Source: CAD feature listing. Evaluate the final solid. Frame: model axes, mm. A direction names the side the tool comes from. Round coordinates to 2 decimals unless told otherwise and drop trailing zeros. Order: outer loops, then holes, each group sorted by start corner. A loop starts at its lowest first (then second) coordinate and runs counter-clockwise, first axis right, second up. Notation, with made-up numbers: M 75.5,-38 L 101.5,-38 A6 ccw 101.5,-28 Z; hole C -28.75,52.25 d5. An arc over 180 degrees is marked long. Use one line per item in the form item = value. Start each with the question number.
Q1. Reachability of faces 1 (the cylindrical face through (-567.96, -22, 0.51)), 2 (the flat face through (-646.372, -29.58, 0.746)), 3 (the flat face through (-8.872, -30.42, 0.746)) from +Z, -Z, +X, -X, +Y, -Y: full face, straight path, thin tool, end or side. Return the list, or none.
Q2. Section D-D (y = -409.5). Return the cut outline in (x, z), plus the area to 3 significant figures.
Q3. Section B-B (x = -577.5). Return the cut outline in (y, z).
Q4. Pull-direction query (X, two-part tool) for faces 4 (the flat face through (10.953, -292.66, 0.246)), 5 (the flat face through (-332, -30, 1)), 6 (the cylindrical face through (-87.49, -24.56, 0.51)), 7 (the cylindrical face through (-78.802, -445.085, 0.507)); classes: pulls with the +X half, pulls with the -X half, needs draft (parallel to the pull), parting line crosses it, or undercut.
Q5. Section A-A (z = 0.85). Return the cut outline in (x, y), plus the area to 3 significant figures.
Q6. Section C-C (y = -25). Return the cut outline in (x, z) (3 decimals).
Q7. Material intervals for probe 1 along Y at (x, z) = (-77.5, 0.2); probe 2 along Y at (x, z) = (-577.5, 0.65); probe 3 along Y at (x, z) = (-37, 0.9), sorted ascending.
from build123d import *

# Parameters (mm, degrees)
F1_DEPTH = 0.5
F3_DEPTH = 0.5
F4_R     = 10
F5_DEPTH = 25


with BuildPart() as f1:
    # F0 (on Top) → F1 (new body)
    with BuildSketch(Plane.XY):
        Polygon((0, 0), (-655, 0), (-687.5, -100), (-645, -480), (-10, -480), (32.5, -100), align=None)
    extrude(amount=F1_DEPTH)

    # F2 (on face) → F3 (join)
    with BuildSketch(Plane.XY.offset(0.5)):
        Polygon((0, 0), (-655, 0), (-637.5, -60), (-17.5, -60), align=None)
        Polygon((-645, -480), (-10, -480), (-17.5, -420), (-637.5, -420), align=None)
    extrude(amount=F3_DEPTH)

    # F4 (on face) → F5 (cut)
    with BuildSketch(Plane.XY.offset(1)):
        with Locations((-577.5, -25)):
            Circle(F4_R)
        with Locations((-577.5, -455)):
            Circle(F4_R)
        with Locations((-77.5, -25)):
            Circle(F4_R)
        with Locations((-77.5, -455)):
            Circle(F4_R)
    extrude(amount=-F5_DEPTH, mode=Mode.SUBTRACT)


solid = f1.part
Results list:
q1.face_1 = +Z, -Z
q1.face_2 = +Z, -X
q1.face_3 = +Z, +X
q2.outline = M -652.88,0 L -2.12,0 L -2.12,0.5 L -652.88,0.5 Z
q2.area = 325 mm2
q3.outline = M -480,0 L -465,0 L -465,1 L -480,1 Z; M -445,0 L -35,0 L -35,1 L -60,1 L -60,0.5 L -420,0.5 L -420,1 L -445,1 Z; M -15,0 L 0,0 L 0,1 L -15,1 Z
q4.face_4 = pulls with the +X half
q4.face_5 = needs draft
q4.face_6 = undercut
q4.face_7 = undercut
q5.outline = M -655,0 L -637.5,-60 L -17.5,-60 L 0,0 Z; M -645,-480 L -10,-480 L -17.5,-420 L -637.5,-420 Z; hole C -577.5,-455 d20; hole C -577.5,-25 d20; hole C -77.5,-455 d20; hole C -77.5,-25 d20
q5.area = 74,600 mm2
q6.outline = M -663.125,0 L -587.5,0 L -587.5,1 L -647.708,1 L -647.708,0.5 L -663.125,0.5 Z; M -567.5,0 L -87.5,0 L -87.5,1 L -567.5,1 Z; M -67.5,0 L 8.125,0 L 8.125,0.5 L -7.292,0.5 L -7.292,1 L -67.5,1 Z
q7.probe_1 = -480 to -465, -445 to -35, -15 to 0
q7.probe_2 = -480 to -465, -445 to -420, -60 to -35, -15 to 0
q7.probe_3 = -480 to -420, -60 to 0
